Read the model definition and answer for the solid it produces. Units are mm, in the model's axes. Coordinates: 2 decimals unless noted, no trailing zeros. Loops run counter-clockwise (first coordinate to the right, second up) from the corner with the lowest first, then second, coordinate; pieces in that order, holes last. Notation, with made-up numbers: (-40, 81) -> (0, 81) arc R38 ccw to (0, 119) -> close; hole circle Ø5 at (4, 52.25). An arc over 180 degrees is marked (long way). Answer in a Markdown table with one row per item.
```python
from build123d import *

# Parameters (mm, degrees)
F1_DEPTH = 5.08
F2_SIZE2 = 2.54
F2_SIZE  = 2.54
F3_W     = 296.9444543123
F3_H     = 473.9504568279
F4_DEPTH = 25.4
F5_DEPTH = 25.4


with BuildPart() as f1:
    # F0 (on Front) → F1 (new body, symmetric)
    with BuildSketch(Plane.XZ):
        with BuildLine():
            Line((-52.1713197231, 34.4429798424), (-58.770544827, 10.8928056434))
            add(Edge.make_bspline(
                [(-58.770544827, 10.8928056434), (-56.5008980701, 12.7169401311), (-52.1836149963, 16.1867774191), (-46.6481737875, 20.7689821181), (-42.103581434, 21.9474441882), (-37.1718262664, 20.3492743447), (-34.4780249811, 18.782172039), (-33.1500247121, 18.009616062)],
                knots=[0, 0, 0, 0, 0.243402605, 0.4629962541, 0.6364782013, 0.8207896592, 1, 1, 1, 1], degree=3))
            Line((-33.1500247121, 18.009616062), (0, 0))
            Line((0, 0), (33.1500247121, 18.009616062))
            add(Edge.make_bspline(
                [(58.770544827, 10.8928056434), (56.5008980701, 12.7169401311), (52.1836149963, 16.1867774191), (46.6481737875, 20.7689821181), (42.103581434, 21.9474441882), (37.1718262664, 20.3492743447), (34.4780249811, 18.782172039), (33.1500247121, 18.009616062)],
                knots=[0, 0, 0, 0, 0.243402605, 0.4629962541, 0.6364782013, 0.8207896592, 1, 1, 1, 1], degree=3))
            Line((58.770544827, 10.8928056434), (52.1713197231, 34.4429798424))
            add(Edge.make_bspline(
                [(52.1713197231, 34.4429798424), (50.9728401731, 36.5972375719), (48.6948112169, 40.6919770164), (44.4995729387, 45.251524036), (40.7511119594, 46.0496576718), (38.4311188014, 45.2100224851), (37.2595414519, 44.7860136628)],
                knots=[0, 0, 0, 0, 0.3036076859, 0.5770871099, 0.7864324897, 1, 1, 1, 1], degree=3))
            Line((37.2595414519, 44.7860136628), (12.3838605359, 31.5890572965))
            add(Edge.make_bspline(
                [(12.3838605359, 31.5890572965), (12.0116389407, 36.4336241706), (11.2801299785, 45.9544153649), (11.9072727509, 59.0755429111), (13.0446244948, 72.3270750889), (15.0430309606, 81.3553880474), (20.0484846376, 98.9141245501), (23.1138356658, 110.0238526226), (25.6900193935, 114.2539658888), (26.796290651, 116.070471704)],
                knots=[0, 0, 0, 0, 0.1554376564, 0.3054740514, 0.451951706, 0.5786332255, 0.7535204728, 0.8941561452, 1, 1, 1, 1], degree=3))
            add(Edge.make_bspline(
                [(26.796290651, 116.070471704), (27.3208616845, 122.376340647), (28.4465148418, 135.9078184294), (30.7430371303, 162.2435359747), (32.8128164069, 193.0751698329), (36.1980689164, 226.214181027), (36.6885878869, 228.6104286649), (36.1789175706, 231.6056884809), (34.578084839, 241.1608396791), (32.1815946616, 268.5632469899), (29.2022062034, 298.3654205907), (26.6745591694, 323.5321383941), (26.2740528758, 332.6532529053), (26.1084791273, 336.424022913)],
                knots=[0, 0, 0, 0, 0.0954552012, 0.2048329812, 0.3319664827, 0.4522041038, 0.4827906265, 0.5164846256, 0.5812786199, 0.6946646008, 0.8165569483, 0.9241626057, 1, 1, 1, 1], degree=3))
            Line((26.1084791273, 336.424022913), (0, 384.5021128654))
            Line((0, 384.5021128654), (-26.1084791273, 336.424022913))
            add(Edge.make_bspline(
                [(-26.796290651, 116.070471704), (-27.3208616845, 122.376340647), (-28.4465148418, 135.9078184294), (-30.7430371303, 162.2435359747), (-32.8128164069, 193.0751698329), (-36.1980689164, 226.214181027), (-36.6885878869, 228.6104286649), (-36.1789175706, 231.6056884809), (-34.578084839, 241.1608396791), (-32.1815946616, 268.5632469899), (-29.2022062034, 298.3654205907), (-26.6745591694, 323.5321383941), (-26.2740528758, 332.6532529053), (-26.1084791273, 336.424022913)],
                knots=[0, 0, 0, 0, 0.0954552012, 0.2048329812, 0.3319664827, 0.4522041038, 0.4827906265, 0.5164846256, 0.5812786199, 0.6946646008, 0.8165569483, 0.9241626057, 1, 1, 1, 1], degree=3))
            add(Edge.make_bspline(
                [(-12.3838605359, 31.5890572965), (-12.0116389407, 36.4336241706), (-11.2801299785, 45.9544153649), (-11.9072727509, 59.0755429111), (-13.0446244948, 72.3270750889), (-15.0430309606, 81.3553880474), (-20.0484846376, 98.9141245501), (-23.1138356658, 110.0238526226), (-25.6900193935, 114.2539658888), (-26.796290651, 116.070471704)],
                knots=[0, 0, 0, 0, 0.1554376564, 0.3054740514, 0.451951706, 0.5786332255, 0.7535204728, 0.8941561452, 1, 1, 1, 1], degree=3))
            Line((-12.3838605359, 31.5890572965), (-37.2595414519, 44.7860136628))
            add(Edge.make_bspline(
                [(-52.1713197231, 34.4429798424), (-50.9728401731, 36.5972375719), (-48.6948112169, 40.6919770164), (-44.4995729387, 45.251524036), (-40.7511119594, 46.0496576718), (-38.4311188014, 45.2100224851), (-37.2595414519, 44.7860136628)],
                knots=[0, 0, 0, 0, 0.3036076859, 0.5770871099, 0.7864324897, 1, 1, 1, 1], degree=3))
        make_face()
    extrude(amount=F1_DEPTH, both=True)

    # F2
    f2_edges = [f1.edges().sort_by_distance(p)[0] for p in [
        (-36.32486, 5.08, 226.315561),
        (-13.693841, 5.08, 74.863456),
        (-24.821701, 5.08, 38.187535),
        (-46.502615, 5.08, 42.946726),
        (-55.470932, 5.08, 22.667893),
        (-47.034517, 5.08, 20.082213),
        (-16.575012, 5.08, 9.004808),
        (16.575012, 5.08, 9.004808),
        (47.034517, 5.08, 20.082213),
        (55.470932, 5.08, 22.667893),
        (46.502615, 5.08, 42.946726),
        (24.821701, 5.08, 38.187535),
        (13.693841, 5.08, 74.863456),
        (36.32486, 5.08, 226.315561),
        (13.05424, 5.08, 360.463068),
        (-13.05424, 5.08, 360.463068),
        (-36.32486, -5.08, 226.315561),
        (-13.693841, -5.08, 74.863456),
        (-24.821701, -5.08, 38.187535),
        (-46.502615, -5.08, 42.946726),
        (-55.470932, -5.08, 22.667893),
        (-47.034517, -5.08, 20.082213),
        (-16.575012, -5.08, 9.004808),
        (16.575012, -5.08, 9.004808),
        (47.034517, -5.08, 20.082213),
        (55.470932, -5.08, 22.667893),
        (46.502615, -5.08, 42.946726),
        (24.821701, -5.08, 38.187535),
        (13.693841, -5.08, 74.863456),
        (36.32486, -5.08, 226.315561),
        (13.05424, -5.08, 360.463068),
        (-13.05424, -5.08, 360.463068),
    ]]
    chamfer(f2_edges, length=F2_SIZE, length2=F2_SIZE2)

    # F3 (on Front) → F4 (cut)
    with BuildSketch(Plane.XZ):
        with Locations((-3.1622722745, 199.3846241385)):
            Rectangle(F3_W, F3_H)
        Polygon((18.1035045534, 120.6582784653), (0, 102.6714965701), (-18.1035045534, 120.6582784653), (-18.1035045534, 331.0994207859), (0, 346.9451367855), (18.1035045534, 331.0994207859), align=None, mode=Mode.SUBTRACT)
    extrude(amount=-F4_DEPTH, mode=Mode.SUBTRACT)

    # F5 (cut): a face of the model
    f5_faces = [f1.faces().sort_by_distance(p)[0] for p in [
        (-9.5209365747, 0, 358.5443317782),
    ]]
    extrude(f5_faces, amount=-F5_DEPTH, mode=Mode.SUBTRACT)


solid = f1.part
```
1. Find the intervals of material crossed by probe 1 along Z at (x, y) = (-6.5, -4); probe 2 along Z at (x, y) = (14.5, 2.25); probe 3 along X at (y, z) = (-0.25, 118), in increasing order.
A:
| item | result |
|---|---|
| probe 1 | z = 109.13 to 341.26 |
| probe 2 | z = 117.08 to 334.25 |
| probe 3 | x = -15.43 to 15.43 |
2. Given pin 1 Ø1.5 at (x, y) = (4, -1) entering from +Z, flat-ended and moving along its own axis, determine where the tip first touches the part or whether it passes through.
A:
| item | result |
|---|---|
| pin 1 | stops at z = 344.1 |
3. A cutting plane is placed at B-B on x = 6.5. Give the vertices of the cut face in (y, z), and give its area (3 significant figures).
A:
| item | result |
|---|---|
| outline | (-5.08, 109.13) -> (5.08, 109.13) -> (5.08, 341.26) -> (-5.08, 341.26) -> close |
| area | 2,360 mm2 |
4. A cutting plane is placed at A-A on y = -1. Give the vertices of the cut face in (x, z).
A:
| item | result |
|---|---|
| outline | (-18.1, 120.66) -> (0, 102.67) -> (18.1, 120.66) -> (18.1, 331.1) -> (0, 346.95) -> (-18.1, 331.1) -> close |
